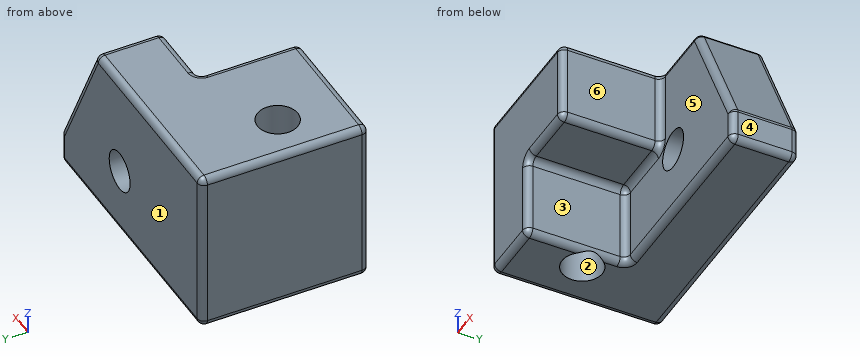
```python
from build123d import *

# Parameters (mm, degrees)
F0_W          = 203.2
F0_H          = 127
F1_DEPTH      = 127
F3_DEPTH      = 76.2
F4_SIZE2      = 101.6
F4_SIZE       = 50.8
F5_R          = 5.08
F6_R          = 15.24
F7_DEPTH      = 101.6
F7_DEPTH_BACK = 101.6
F8_R          = 15.24
F9_DEPTH      = 127
F9_DEPTH_BACK = 127


with BuildPart() as f1:
    # F0 (on Front) → F1 (new body)
    with BuildSketch(Plane.XZ):
        Rectangle(F0_W, F0_H)
    extrude(amount=F1_DEPTH)

    # F2 (on face) → F3 (cut)
    with BuildSketch(Plane.XZ.offset(127)):
        Polygon((101.6, 63.5), (0, 63.5), (0, 0), (-50.8298836648, 0), (-50.8298836648, -63.5), (101.6, -63.5), align=None)
    extrude(amount=-F3_DEPTH, mode=Mode.SUBTRACT)

    # F4
    f4_edges = [f1.edges().sort_by_distance(p)[0] for p in [
        (101.6, -25.4, 63.5),
    ]]
    f4_side = f1.faces().sort_by_distance((-21.771429, -52.614286, 63.5))[0]
    chamfer(f4_edges, length=F4_SIZE, length2=F4_SIZE2, reference=f4_side)

    # F5
    f5_edges = [f1.edges().sort_by_distance(p)[0] for p in [
        (-25.4, 0, 63.5),
        (50.8, -25.4, 63.5),
        (-101.6, -63.5, 63.5),
        (25.4, -50.8, 63.5),
        (-50.8, -127, 63.5),
        (0, -88.9, 63.5),
        (-76.214942, -127, -63.5),
        (-101.6, -127, 0),
        (0, -127, 31.75),
        (-25.414942, -127, 0),
        (-50.829884, -127, -31.75),
        (0, -88.9, 0),
        (0, -50.8, 31.75),
        (-50.829884, -88.9, 0),
        (-50.829884, -88.9, -63.5),
        (-50.829884, -50.8, -31.75),
        (76.2, -50.8, 12.7),
        (101.6, -50.8, -50.8),
        (-25.414942, -50.8, 0),
        (25.385058, -50.8, -63.5),
        (76.2, 0, 12.7),
        (101.6, -25.4, -38.1),
        (101.6, 0, -50.8),
        (101.6, -25.4, -63.5),
        (-101.6, -63.5, -63.5),
        (-101.6, 0, 0),
        (0, 0, -63.5),
    ]]
    fillet(f5_edges, radius=F5_R)

    # F6 (on face) → F7 (cut, two sides)
    with BuildSketch(Plane.XZ.offset(50.8)) as f7_sk:
        with Locations((16.4750218391, -12.237187475)):
            Circle(F6_R)
    extrude(amount=-F7_DEPTH, mode=Mode.SUBTRACT)
    extrude(f7_sk.sketch, amount=F7_DEPTH_BACK, mode=Mode.SUBTRACT)

    # F8 (on face) → F9 (cut, two sides)
    with BuildSketch(Plane.XY.offset(63.5)) as f9_sk:
        with Locations((-66.8318793178, -76.2298852205)):
            Circle(F8_R)
    extrude(amount=F9_DEPTH, mode=Mode.SUBTRACT)
    extrude(f9_sk.sketch, amount=-F9_DEPTH_BACK, mode=Mode.SUBTRACT)


solid = f1.part
```
Verification items for the finished model (mm, model axes). Face numbers are marked on the shaded views. A direction names the side the tool comes from. Coordinates: 2 decimals unless noted, no trailing zeros. Loops run counter-clockwise (first coordinate to the right, second up) from the corner with the lowest first, then second, coordinate; pieces in that order, holes last. Notation, with made-up numbers: (-25, -3) - (-5, -3) arc R32 cw to (-5, 33) - close; hole circle Ø4 at (47, 29). An arc over 180 degrees is marked (long way). Return JSON: item names as keys, results as strings.
1. Mould release check, pull along X, two halves, no side actions. Record for the marked faces 1, 2 and 3: +X half, -X half, draft (parallel to the pull), parting line (faces both ways), or undercut.
Established:
{"face 1": "draft", "face 2": "undercut", "face 3": "+X half"}
2. Go/stop test with flat-tipped pins: pin 1 (2 mm diameter, centred on y = -106, z = 8.5, fed in from +X); pin 2 (5 mm diameter, centred on x = 17.5, z = 27, fed in from -Y); pin 3 (1.5 mm diameter, centred on y = -32.5, z = -28.5, fed in from +X) (3 decimals). Record where each tip stops, or that it passes through.
Established:
{"pin 1": "stops at x = 0", "pin 2": "stops at y = -50.8", "pin 3": "stops at x = 97.175"}
3. Thickness scan on L1, parallel to Y at x = 15.5, z = -32; L2, parallel to X at y = -37.5, z = -1.5; L3, parallel to X at y = -76, z = -58. Record the ranges inside material, lowest first.
Established:
{"L1": "y = -50.8 to 0", "L2": "x = -101.6 to 5.66, 27.29 to 83.3", "L3": "x = -101.6 to -82.07, -51.59 to -50.83"}
4. Section check A-A, the plane y = -70. Record the boundary of the cut face in (x, z).
Established:
{"outline": "(-101.6, -58.42) arc R5.08 ccw to (-96.52, -63.5) - (-80.74, -63.5) - (-80.74, 63.5) - (-96.52, 63.5) arc R5.08 ccw to (-101.6, 58.42) - close; (-52.92, -62.53) arc R5.08 ccw to (-50.83, -58.42) - (-50.83, -5.08) arc R5.08 cw to (-45.75, 0) - (-5.08, 0) arc R5.08 ccw to (0, 5.08) - (0, 58.42) arc R5.08 ccw to (-5.08, 63.5) - (-52.92, 63.5) - close"}
5. Section check C-C, the plane y = -118. Record the boundary of the cut face in (x, z), then the cut area to 3 significant figures.
Established:
{"outline": "(-101.6, -58.42) arc R5.08 ccw to (-96.52, -63.5) - (-55.91, -63.5) arc R5.08 ccw to (-50.83, -58.42) - (-50.83, -5.08) arc R5.08 cw to (-45.75, 0) - (-5.08, 0) arc R5.08 ccw to (0, 5.08) - (0, 58.42) arc R5.08 ccw to (-5.08, 63.5) - (-96.52, 63.5) arc R5.08 ccw to (-101.6, 58.42) - close", "area": "9,650 mm2"}
6. Section check B-B, the plane x = -62. Record the boundary of the cut face in (y, z), then the cut area to 3 significant figures.
Established:
{"outline": "(-127, -58.42) arc R5.08 ccw to (-121.92, -63.5) - (-90.68, -63.5) - (-90.68, 63.5) - (-121.92, 63.5) arc R5.08 ccw to (-127, 58.42) - close; (-61.78, -63.5) - (-5.08, -63.5) arc R5.08 ccw to (0, -58.42) - (0, 58.42) arc R5.08 ccw to (-5.08, 63.5) - (-61.78, 63.5) - close", "area": "12,400 mm2"}
7. Tool access check on the marked faces 4, 5 and 6. Record the directions out of +Z, -Z, +X, -X, +Y, -Y that give a thin tool (end or side, any length) a straight path to the whole face; none if there is none.
Established:
{"face 4": "+Z, -Z, +X, +Y, -Y", "face 5": "-Z, +X, -Y", "face 6": "+Z, -Z, +X, -Y"}
8. Section check D-D, the plane x = -33. Record the boundary of the cut face in (y, z).
Established:
{"outline": "(-127, 5.08) arc R5.08 ccw to (-121.92, 0) - (-55.88, 0) arc R5.08 cw to (-50.8, -5.08) - (-50.8, -58.42) arc R5.08 ccw to (-45.72, -63.5) - (-5.08, -63.5) arc R5.08 ccw to (0, -58.42) - (0, 58.42) arc R5.08 ccw to (-5.08, 63.5) - (-121.92, 63.5) arc R5.08 ccw to (-127, 58.42) - close"}
